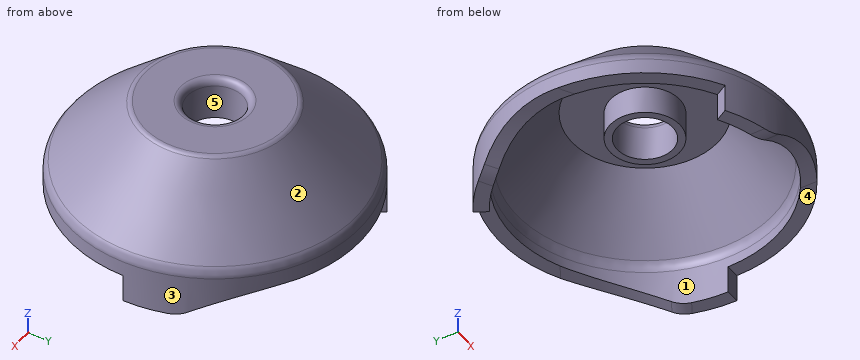
```python
from build123d import *

# Parameters (mm, degrees)
ESQUISSE1_R                  = 5
ESQUISSE1_R_2                = 4
BASE_EXTRUSION_DEPTH         = 4
ESQUISSE2_R                  = 10.5
ESQUISSE2_R_2                = 4
BOSS_EXTRU_1_DEPTH           = 2
ENL_V_MAT_EXTRU_1_DEPTH      = 32.670175244
R_P_TITION_CIRCULAIRE1_COUNT = 3
CONG_1_R                     = 5
CONG_2_R                     = 1


with BuildPart() as part:
    # Esquisse1 → Base-Extrusion (new body)
    with BuildSketch(Plane.XY):
        Circle(ESQUISSE1_R)
        Circle(ESQUISSE1_R_2, mode=Mode.SUBTRACT)
    extrude(amount=BASE_EXTRUSION_DEPTH)

    # Esquisse2 → Boss.-Extru.1 (add)
    with BuildSketch(Plane.XY.offset(4)):
        Circle(ESQUISSE2_R)
        Circle(ESQUISSE2_R_2, mode=Mode.SUBTRACT)
    extrude(amount=BOSS_EXTRU_1_DEPTH)

    # Esquisse3 → Boss.-R_vol.1 (revolve)
    with BuildSketch(Plane(origin=(0, 0, 0), x_dir=(1, 0, 0), z_dir=(0, 1, 0))):
        with BuildLine():
            Line((-10.5, -6), (-20.379310345, 3.408866995))
            ThreePointArc((-20.379310345, 3.408866995), (-20.83829006, 4.06930426), (-21, 4.857142857))
            Line((-21, 4.857142857), (-21, 6))
            Line((-21, 6), (-21, 11))
            Line((-21, 11), (-19, 11))
            Line((-19, 11), (-19, 5.5))
            ThreePointArc((-19, 5.5), (-18.851832131, 4.744541358), (-18.429282241, 4.101017414))
            Line((-18.429282241, 4.101017414), (-10.5, -4))
            Line((-10.5, -4), (-10.5, -6))
        make_face()
    revolve(axis=Axis((0, 0, -19.062079538), (0, 0, 1)))

    # Esquisse4 → Enl_v. mat.-Extru.1 (cut, through all)
    with BuildSketch(Plane(origin=(0, 0, 0), x_dir=(1, 0, 0), z_dir=(0, 1, 0))):
        with BuildLine():
            Line((11.003277804, 7.020139439), (23.595787982, 7.020139439))
            Line((23.595787982, 7.020139439), (23.595787982, 11.020139439))
            ThreePointArc((23.595787982, 11.020139439), (2.431434716, 55.826808841), (11.003277804, 7.020139439))
        make_face()
    enl_v_mat_extru_1 = extrude(amount=-ENL_V_MAT_EXTRU_1_DEPTH, mode=Mode.SUBTRACT)

    # R_p_tition circulaire1: Enl_v. mat.-Extru.1 ×3 about axis
    r_p_tition_circulaire1_axis = Axis((0, 0, 0), (0, 0, 1))
    for i in range(1, R_P_TITION_CIRCULAIRE1_COUNT):
        add(enl_v_mat_extru_1.rotate(r_p_tition_circulaire1_axis, i * 360 / R_P_TITION_CIRCULAIRE1_COUNT), mode=Mode.SUBTRACT)

    # Cong_1
    cong_1_edges = [part.edges().sort_by_distance(p)[0] for p in [
        (-15.260123677, 12.926551295, -11),
        (-3.564659966, -19.678930416, -11),
        (18.824783643, 6.752379122, -11),
    ]]
    fillet(cong_1_edges, radius=CONG_1_R)

    # Cong_2
    cong_2_edges = [part.edges().sort_by_distance(p)[0] for p in [
        (10.5, 0, 6),
        (-4, 0, 6),
    ]]
    fillet(cong_2_edges, radius=CONG_2_R)


solid = part.part
```
Design review of the part built by this model. Coordinates are the model's own, in mm. Face numbers are marked on the shaded views. A direction names the side the tool comes from. Coordinates: 2 decimals unless noted, no trailing zeros. Order: outer loops, then holes, each group sorted by start corner. A loop starts at its lowest first (then second) coordinate and runs counter-clockwise, first axis right, second up. Notation, with made-up numbers: (15.25, -17) - (19.25, -17) arc R18 ccw to (19.25, 17) - close; hole circle Ø3 at (41, 36.25). An arc over 180 degrees is marked (long way). Answer in a Markdown table with one row per item.
(1) Consider section A-A on x = 0. State the section outline as (y, z) points.
Checked values:
| item | result |
|---|---|
| outline | (-21, -9.09) - (-19, -9.09) - (-19, -5.5) arc R2 cw to (-18.43, -4.1) - (-10.5, 4) - (-5, 4) - (-5, 0) - (-4, 0) - (-4, 5) arc R1 ccw to (-5, 6) - (-10.1, 6) arc R1 ccw to (-10.79, 5.72) - (-20.38, -3.41) arc R2 ccw to (-21, -4.86) - close; (4, 0) - (5, 0) - (5, 4) - (10.5, 4) - (18.43, -4.1) arc R2 cw to (19, -5.5) - (19, -7.02) - (21, -7.02) - (21, -4.86) arc R2 ccw to (20.38, -3.41) - (10.79, 5.72) arc R1 ccw to (10.1, 6) - (5, 6) arc R1 ccw to (4, 5) - close |
(2) Wall thickness on line 1 along Y through (x, z) = (0, -6.8); line 2 along Y through (x, z) = (0, 2.9) (3 decimals); line 3 along Y through (x, z) = (14, -6.75): over which ranges is each line inside the solid? List them lowest first. Write a range as from..to.
Checked values:
| item | result |
|---|---|
| line 1 | -21..-19, 19..21 |
| line 2 | -13.755..-11.577, -5..-4, 4..5, 11.577..13.755 |
| line 3 | -15.65..-12.85, 12.85..15.65 |
(3) The part is to be moulded in two halves that separate along Y. For the marked faces 3, 4 and 5, say which applies: released by +Y, released by -Y, zero draft, split by the parting line, or undercut.
Checked values:
| item | result |
|---|---|
| face 3 | split by the parting line |
| face 4 | zero draft |
| face 5 | undercut |
(4) Clearance check with flat-ended pins moving along their axes: pin 1 (2 mm diameter, centred on x = 16, z = -6.5, fed in from +Y); pin 2 (2 mm diameter, centred on y = 13, z = -7.5, fed in from +X); pin 3 (3.5 mm diameter, centred on x = 2.5, y = 19, fed in from -Z). State where each tip first meets the part, or that it passes through.
Checked values:
| item | result |
|---|---|
| pin 1 | y = 14.7 |
| pin 2 | x = 17.23 |
| pin 3 | z = -7.02 |
(5) For the marked faces 1 and 2, list the 3-axis set-ups (+Z, -Z, +X, -X, +Y, -Y) from which the entire face can be reached by the end or side of a thin tool; tool diameter is ignored.
Checked values:
| item | result |
|---|---|
| face 1 | -Z |
| face 2 | +Z |
